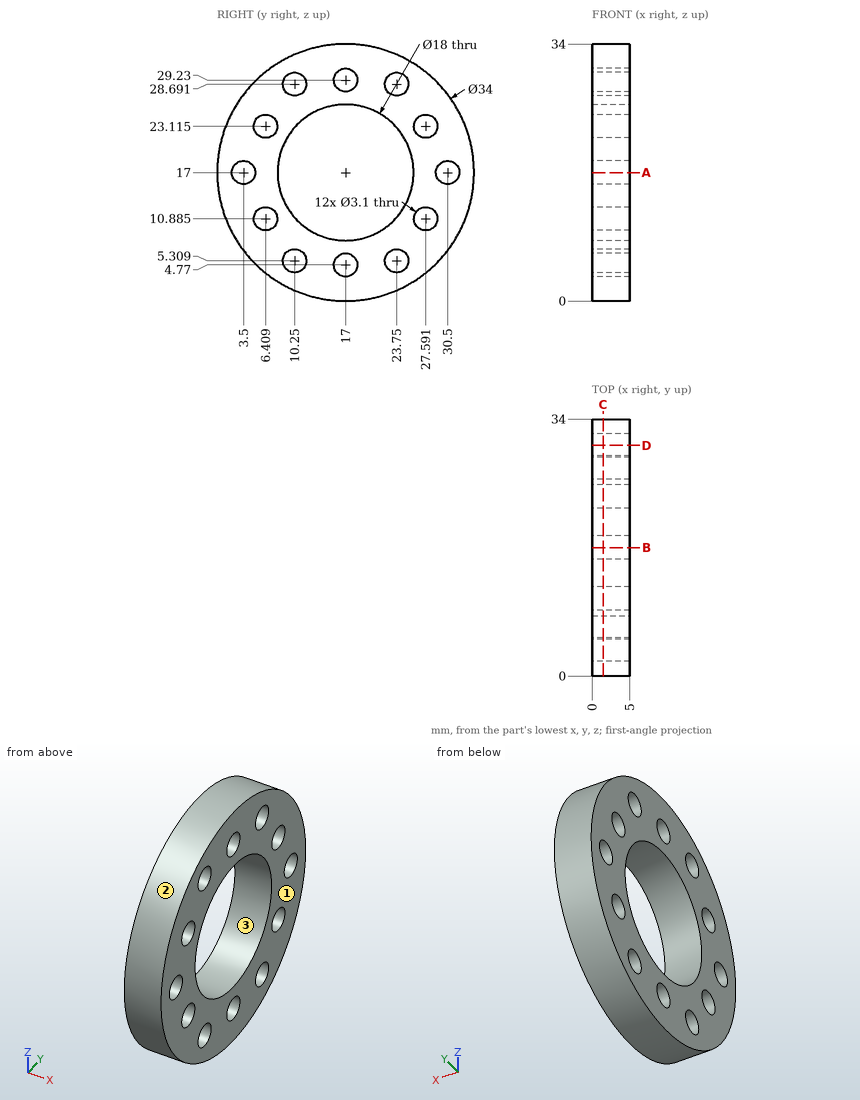
Here's the drawing with two shaded views (mm, measured from the low corner). I have some questions. Give positions to 0.01 mm unless a question says otherwise; leave off trailing zeros. Order: outer loops, then holes, each group sorted by start corner. A loop starts at its lowest first (then second) coordinate and runs counter-clockwise, first axis right, second up. Notation, with made-up numbers: M 79.25,-13 L 114.25,-13 A6 ccw 114.25,-6 Z; hole C 65.25,23.5 d6. An arc over 180 degrees is marked long. One line per question, with ' | ' between items.
Item 1: I'm going to push flat-ended pins straight in: pin 1 Ø1 at (x, y) = (3, 7.5) entering from -Z; pin 2 Ø2 at (x, z) = (4, 18) entering from -Y; pin 3 Ø2 at (x, z) = (4.5, 8) entering from +Y; pin 4 Ø3 at (x, z) = (1, 12) entering from +Y (1 decimal). Where does each tip first touch, or does it pass through?
Answer block:
pin 1: stops at z = 2.58 | pin 2: stops at y = 0 | pin 3: stops at y = 32 | pin 4: stops at y = 33.6
Item 2: Suppose I cut it at A-A, the plane z = 17. Write out the boundary of the cut face in (x, y).
Answer block:
outline: M 0,0 L 5,0 L 5,1.95 L 0,1.95 Z; M 0,5.05 L 5,5.05 L 5,8 L 0,8 Z; M 0,26 L 5,26 L 5,28.95 L 0,28.95 Z; M 0,32.05 L 5,32.05 L 5,34 L 0,34 Z
Item 3: Suppose I cut it at D-D, the plane y = 30.5. Write out the boundary of the cut face in (x, z).
Answer block:
outline: M 0,6.67 L 5,6.67 L 5,15.45 L 0,15.45 Z; M 0,18.55 L 5,18.55 L 5,27.33 L 0,27.33 Z
Item 4: Suppose I cut it at C-C, the plane x = 1.45. Give the number of separate pieces and of enclosed holes in the cut face, then the cut area to 3 significant figures.
Answer block:
separate pieces: 1 | enclosed holes: 13 | area: 563 mm2
Item 5: Suppose I cut it at B-B, the plane y = 17. Write out the boundary of the cut face in (x, z).
Answer block:
outline: M 0,0 L 5,0 L 5,3.22 L 0,3.22 Z; M 0,6.32 L 5,6.32 L 5,8 L 0,8 Z; M 0,26 L 5,26 L 5,27.68 L 0,27.68 Z; M 0,30.78 L 5,30.78 L 5,34 L 0,34 Z
Item 6: We'd pull the mould along Z, two halves only. Please class the marked faces 1, 2 and 3: released by +Z, released by -Z, zero draft, split by the parting line, or undercut.
Answer block:
face 1: zero draft | face 2: split by the parting line | face 3: undercut
Item 7: Please list where these lines run through material, in increasing order: L1, parallel to Y at x = 3.15, z = 28 (1 decimal); L2, parallel to Y at x = 0.75, z = 27.5 (1 decimal); L3, parallel to Y at x = 2.7, z = 10 (1 decimal).
Answer block:
L1: y = 4 to 8.9, 11.6 to 16.1, 17.9 to 22.4, 25.1 to 30 | L2: y = 3.6 to 9.3, 11.2 to 22.8, 24.7 to 30.4 | L3: y = 1.5 to 5.1, 7.7 to 11.3, 22.7 to 26.3, 28.9 to 32.5
